Source: three-view drawing plus pictorial views. Frame: mm from the lowest corner of the part. A direction names the side the tool comes from. Give positions to 0.01 mm unless a question says otherwise; leave off trailing zeros. Order: outer loops, then holes, each group sorted by start corner. A loop starts at its lowest first (then second) coordinate and runs counter-clockwise, first axis right, second up. Notation, with made-up numbers: (26.5, 60) - (71.5, 60) arc R31 ccw to (71.5, 94) - close; hole circle Ø1 at (20, -16). An arc over 180 degrees is marked (long way). Answer in a Markdown table with one row per item. Add a question column.
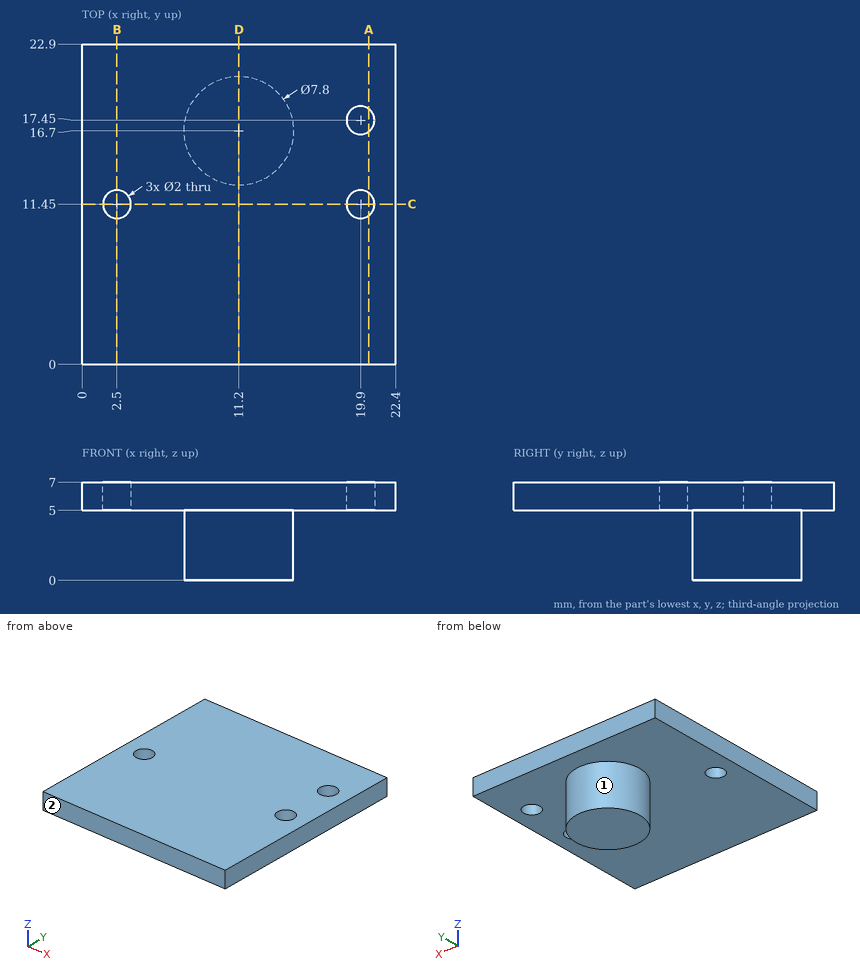
Q1. Contact query for flat-ended pins moving along their axis: P1, Ø5, axis at x = 6, y = 6.5, coming from the -Z side; P2, Ø1.5, axis at y = 14, z = 3.5, coming from the -X side; P3, Ø11, axis at x = 13.5, y = 14, coming from the -Z side; P4, Ø1.8, axis at x = 2.5, y = 11.45, coming from the +Z side. Output: stop coordinate, or through.
Q2. Section D-D, the plane x = 11.2. Return loops of the section in (y, z).
Q3. Section A-A, the plane x = 20.5. Return loops of the section in (y, z).
Q4. Section C-C, the plane y = 11.45. Return loops of the section in (x, z), then the cut area to 3 significant figures.
Q5. Access query for the marked faces 1 and 2. Directions: +Z, -Z, +X, -X, +Y, -Y. A direction counts if a zero-diameter tool reaches every point of the face in a straight line with its end or side. Return the directions, or none.
Q6. Line query: probe 1 along Y at (x, z) = (19.9, 6.05); probe 2 along Y at (x, z) = (2.5, 6.25); probe 3 along Z at (x, y) = (18, 2). Output: solid intervals per line, ascending.
Q7. Section B-B, the plane x = 2.5. Return loops of the section in (y, z), then the cut area to 3 significant figures.
Computed:
| question | item | result |
|---|---|---|
| 1 | P1 | stops at z = 5 |
| 1 | P2 | stops at x = 7.82 |
| 1 | P3 | stops at z = 0 |
| 1 | P4 | passes through |
| 2 | outline | (0, 5) - (12.8, 5) - (12.8, 0) - (20.6, 0) - (20.6, 5) - (22.9, 5) - (22.9, 7) - (0, 7) - close |
| 3 | outline | (0, 5) - (10.65, 5) - (10.65, 7) - (0, 7) - close; (12.25, 5) - (16.65, 5) - (16.65, 7) - (12.25, 7) - close; (18.25, 5) - (22.9, 5) - (22.9, 7) - (18.25, 7) - close |
| 4 | outline | (0, 5) - (1.5, 5) - (1.5, 7) - (0, 7) - close; (3.5, 5) - (18.9, 5) - (18.9, 7) - (3.5, 7) - close; (20.9, 5) - (22.4, 5) - (22.4, 7) - (20.9, 7) - close |
| 4 | area | 36.8 mm^2 |
| 5 | face 1 | -Z |
| 5 | face 2 | +Z, -Z, +X, -X, -Y |
| 6 | probe 1 | y = 0 to 10.45, 12.45 to 16.45, 18.45 to 22.9 |
| 6 | probe 2 | y = 0 to 10.45, 12.45 to 22.9 |
| 6 | probe 3 | z = 5 to 7 |
| 7 | outline | (0, 5) - (10.45, 5) - (10.45, 7) - (0, 7) - close; (12.45, 5) - (22.9, 5) - (22.9, 7) - (12.45, 7) - close |
| 7 | area | 41.8 mm^2 |
